Verification items for the finished model (mm, model axes). Face numbers are marked on the shaded views. A direction names the side the tool comes from. Round coordinates to 2 decimals unless told otherwise and drop trailing zeros. Write each loop counter-clockwise with the first axis right and the second up, starting at its lowest first coordinate (ties: lowest second). Pieces come first, ordered by that corner, then holes. Notation, with made-up numbers: (58.25, 76) -> (116.25, 76) arc R16 cw to (116.25, 80) -> close; hole circle Ø5 at (86, -12.75). An arc over 180 degrees is marked (long way). Answer as a JSON object with one key per item and string values. Group by question number.
(1) Sectioned sample at D-D on y = 13. Record the cut outline in (x, z), and give its area (3 significant figures).
(2) Set-up check for the marked faces 4, 5 and 6: record each of +Z, -Z, +X, -X, +Y, -Y from which the full face is reachable in a straight line by a thin tool's end or side.
(3) Sectioned sample at A-A on x = 0. Record the cut outline in (y, z), and give its area (3 significant figures).
(4) Draft check along X on the marked faces 1, 2 and 3. Enter one of: released by +X, released by -X, zero draft, split by the parting line, or undercut.
(5) Sectioned sample at C-C on y = 2. Record the cut outline in (x, z), and give its area (3 significant figures).
(6) Gauge pin test, flat ends, axial feed: pin 1 Ø4.5 at (x, z) = (18.5, 4.5) entering from +Y; pin 2 Ø3 at (y, z) = (-2, 5) entering from +X; pin 3 Ø2 at (x, z) = (-4, 5) entering from +Y. Record the tip position at first contact, or that the pin passes through.
(7) Sectioned sample at B-B on z = 5. Record the cut outline in (x, y), and give its area (3 significant figures).
(8) Scan lines: L1, parallel to Y at x = 0, z = 6.25; L2, parallel to X at y = 3, z = 5; L3, parallel to X at y = -0.75, z = 5. Record each from-to range of solid material in increasing order. Write a range as from..to.
```python
from build123d import *

# Parameters (mm, degrees)
SALIENTE_EXTRUIR1_DEPTH    = 10
CROQUIS2_W                 = 24.660026533
CROQUIS2_H                 = 3
SALIENTE_EXTRUIR2_DEPTH    = 15
CORTAR_EXTRUIR1_DEPTH      = 15
REDONDEO1_R                = 2
CROQUIS4_R                 = 1.75
CORTAR_EXTRUIR2_DEPTH      = 15
CORTAR_EXTRUIR2_DEPTH_BACK = 25
CROQUIS5_R                 = 2.5
CORTAR_EXTRUIR3_DEPTH      = 25
CORTAR_EXTRUIR4_DEPTH      = 25


with BuildPart() as part:
    # Croquis1 → Saliente-Extruir1 (new body)
    with BuildSketch(Plane.XY):
        with BuildLine():
            Line((-17.688572934, 0), (-17.688572934, -17.5))
            Line((-17.688572934, -17.5), (16.971453599, -17.5))
            Line((16.971453599, -17.5), (16.971453599, -3.5))
            Line((16.971453599, -3.5), (20.971453599, -3.5))
            Line((20.971453599, -3.5), (20.971453599, 0))
            Line((20.971453599, 0), (13.5, 0))
            ThreePointArc((13.5, 0), (-13.494189444, -0.396044516), (13.476762776, 0.791748108))
            Line((13.476762776, 0.791748108), (21.160026533, 0.791748108))
            Line((21.160026533, 0.791748108), (21.160026533, 4.291748108))
            Line((21.160026533, 4.291748108), (17.160026533, 4.291748108))
            ThreePointArc((17.160026533, 4.291748108), (-2.162085979, 17.555939071), (-17.688572934, 0))
        make_face()
    extrude(amount=SALIENTE_EXTRUIR1_DEPTH)

    # Croquis2 → Saliente-Extruir2 (add)
    with BuildSketch(Plane(origin=(0, 0, 0), x_dir=(-1, 0, 0), z_dir=(0, 0, -1))):
        with Locations((0.358559668, -16)):
            Rectangle(CROQUIS2_W, CROQUIS2_H)
    extrude(amount=SALIENTE_EXTRUIR2_DEPTH)

    # Croquis3 → Cortar-Extruir1 (cut)
    with BuildSketch(Plane.XZ.offset(17.5)):
        with BuildLine():
            Line((5.811427066, -6.5), (5.811427066, -11.5))
            ThreePointArc((5.811427066, -11.5), (4.811427066, -12.5), (3.811427066, -11.5))
            Line((3.811427066, -11.5), (3.811427066, -6.5))
            ThreePointArc((3.811427066, -6.5), (4.811427066, -5.5), (5.811427066, -6.5))
        make_face()
        with BuildLine():
            Line((-4.188572934, -6.5), (-4.188572934, -11.5))
            ThreePointArc((-4.188572934, -11.5), (-5.188572934, -12.5), (-6.188572934, -11.5))
            Line((-6.188572934, -11.5), (-6.188572934, -6.5))
            ThreePointArc((-6.188572934, -6.5), (-5.188572934, -5.5), (-4.188572934, -6.5))
        make_face()
    extrude(amount=-CORTAR_EXTRUIR1_DEPTH, mode=Mode.SUBTRACT)

    # Redondeo1
    redondeo1_edges = [part.edges().sort_by_distance(p)[0] for p in [
        (16.971453599, -17.5, 5),
        (-17.688572934, -17.5, 5),
        (11.971453599, -16, -15),
        (-12.688572934, -16, -15),
        (21.160026533, 2.541748108, 10),
        (20.971453599, -1.75, 10),
        (20.971453599, -1.75, 0),
        (21.160026533, 2.541748108, 0),
    ]]
    fillet(redondeo1_edges, radius=REDONDEO1_R)

    # Croquis4 → Cortar-Extruir2 (cut, two sides)
    with BuildSketch(Plane(origin=(0, 4.291748108, 0), x_dir=(1, 0, 0), z_dir=(0, 1, 0))) as cortar_extruir2_sk:
        with Locations((17.857152829, -5)):
            Circle(CROQUIS4_R)
    extrude(amount=CORTAR_EXTRUIR2_DEPTH, mode=Mode.SUBTRACT)
    extrude(cortar_extruir2_sk.sketch, amount=-CORTAR_EXTRUIR2_DEPTH_BACK, mode=Mode.SUBTRACT)

    # Croquis5 → Cortar-Extruir3 (cut)
    with BuildSketch(Plane(origin=(0, 4.291748108, 0), x_dir=(1, 0, 0), z_dir=(0, 1, 0))):
        with Locations((17.857152829, -5)):
            Circle(CROQUIS5_R)
    extrude(amount=CORTAR_EXTRUIR3_DEPTH, mode=Mode.SUBTRACT)

    # Croquis8 → Cortar-Extruir4 (cut)
    with BuildSketch(Plane.XZ.offset(3.5)):
        Polygon((17.857152829, 7.937414178), (15.313277529, 6.468707089), (15.313277529, 3.531292911), (17.857152829, 2.062585822), (20.401028129, 3.531292911), (20.401028129, 6.468707089), align=None)
    extrude(amount=CORTAR_EXTRUIR4_DEPTH, mode=Mode.SUBTRACT)


solid = part.part
```
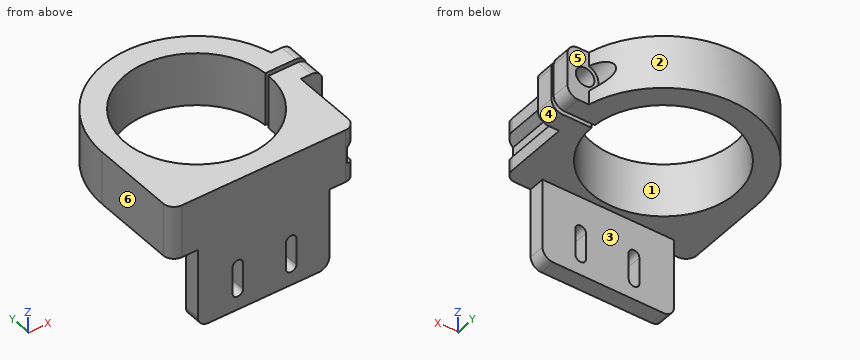
Computed values:
{
 "1": {"outline": "(-12, 0) -> (-3.64, 0) -> (-3.64, 10) -> (-12, 10) -> close; (3.64, 0) -> (12, 0) -> (12, 10) -> (3.64, 10) -> close", "area": "167 mm2"},
 "2": {"face 4": "-Z, +X, -Y", "face 5": "+X, +Y", "face 6": "+Z, -Z, -X, +Y, -Y"},
 "3": {"outline": "(-17.5, -15) -> (-14.5, -15) -> (-14.5, 0) -> (-13.5, 0) -> (-13.5, 10) -> (-17.5, 10) -> close; (13.5, 0) -> (17.69, 0) -> (17.69, 10) -> (13.5, 10) -> close", "area": "127 mm2"},
 "4": {"face 1": "undercut", "face 2": "split by the parting line", "face 3": "zero draft"},
 "5": {"outline": "(-17.58, 0) -> (-13.35, 0) -> (-13.35, 10) -> (-17.58, 10) -> close; (13.35, 0) -> (19.16, 0) arc R2 ccw to (21.16, 2) -> (21.16, 8) arc R2 ccw to (19.16, 10) -> (13.35, 10) -> close; hole circle Ø3.5 at (17.86, 5)", "area": "109 mm2"},
 "6": {"pin 1": "y = 4.29", "pin 2": "x = 20.97", "pin 3": "y = 17.43"},
 "7": {"outline": "(-17.69, -15.5) arc R2 ccw to (-15.69, -17.5) -> (14.97, -17.5) arc R2 ccw to (15.31, -17.47) -> (15.31, -3.5) -> (16.11, -3.5) -> (16.11, 0) -> (13.5, 0) arc R13.5 cw (long way) to (13.48, 0.79) -> (16.11, 0.79) -> (16.11, 4.29) -> (15.36, 4.29) -> (15.36, 8.78) arc R17.69 ccw to (-17.69, 0) -> close; (19.61, -3.5) -> (20.97, -3.5) -> (20.97, 0) -> (19.61, 0) -> close; (19.61, 0.79) -> (21.16, 0.79) -> (21.16, 4.29) -> (19.61, 4.29) -> close", "area": "496 mm2"},
 "8": {"L1": "-17.5..-13.5, 13.5..17.69", "L2": "-17.43..-13.16, 13.16..16.11, 19.61..21.16", "L3": "-17.69..-13.48, 13.48..16.11, 19.61..20.97"}
}
